from build123d import *

# Parameters (mm, degrees)
F0_R     = 20
F1_DEPTH = 5
F2_R     = 5
F3_DEPTH = 75
F4_R     = 4
F5_DEPTH = 3
F6_SIZE2 = 1
F6_SIZE  = 0.25
F7_R     = 4.99999
F9_D     = 2.75
F9_DEPTH = 7
F9_TIP   = 0.8261833512


# Not quite as in the source:
# - a fillet or chamfer is up to 0.001 mm smaller than in the source, because OpenCascade refuses the exact size


with BuildPart() as f1:
    # F0 (on Top) → F1 (new body)
    with BuildSketch(Plane.XY):
        Circle(F0_R)
    extrude(amount=F1_DEPTH)

    # F2 (on face) → F3 (join)
    with BuildSketch(Plane.XY.offset(5)):
        Circle(F2_R)
    extrude(amount=F3_DEPTH)

    # F4 (on face) → F5 (join)
    with BuildSketch(Plane.XY.offset(80)):
        Circle(F4_R)
    extrude(amount=F5_DEPTH)

    # F6
    f6_edges = [f1.edges().sort_by_distance(p)[0] for p in [
        (-4, 0, 83),
    ]]
    f6_side = f1.faces().sort_by_distance((0, 0, 83))[0]
    chamfer(f6_edges, length=F6_SIZE, length2=F6_SIZE2, reference=f6_side)

    # F7 (radius 5 in the source; OpenCascade refuses exactly that, so slightly less here)
    f7_edges = [f1.edges().sort_by_distance(p)[0] for p in [
        (-20, 0, 5),
        (-5, 0, 5),
    ]]
    fillet(f7_edges, radius=F7_R)

    # F9
    with Locations(Plane.XY.offset(83)):
        with Locations((0, 0)):
            Hole(F9_D / 2, depth=F9_DEPTH)
            with Locations((0, 0, -(F9_DEPTH + F9_TIP / 2))):  # 118° drill point
                Cone(0, F9_D / 2, F9_TIP, mode=Mode.SUBTRACT)


solid = f1.part
CAD build for the part. Positions are in the model's coordinates, mm. A direction names the side the tool comes from. Round coordinates to 2 decimals unless told otherwise and drop trailing zeros. Write each loop counter-clockwise with the first axis right and the second up, starting at its lowest first coordinate (ties: lowest second). Pieces come first, ordered by that corner, then holes. Notation, with made-up numbers: M -22.5,73 L 33.5,73 A17 ccw 33.5,89 Z; hole C 85.25,5.25 d7. An arc over 180 degrees is marked long. Put each result on its own line as item: value. Start each with the question number.
1) Pin check, flat tips, straight feed: pin 1 Ø8 at (x, z) = (-10.5, 36.5) entering from +Y; pin 2 Ø3 at (x, z) = (-3.5, 51) entering from +Y; pin 3 Ø1 at (x, y) = (8.5, -15.5) entering from +Z; pin 4 Ø10 at (x, y) = (9, -2.5) entering from +Z. Stop position of each tip, or through.
2) Drill centre lines: probe 1 along Y at (x, z) = (0, 78.5) (3 decimals); probe 2 along Z at (x, y) = (-7, -13); probe 3 along Y at (x, z) = (0, 81) (3 decimals). Where is each one in solid material? Low to high. Write a range as [from, to].
3) Saw through at A-A, the plane z = 36. Write the cut outline in (x, y).
4) Pull direction X, two halves, no side cores. Call faces 3 (the conical face through (0.23, 0.07, 75.32)), 4 (the cylindrical face through (-1.08, -4.88, 44.51)), 5 (the flat face through (0, 0, 0)), 6 (the cylindrical face through (0.3, -1.34, 79.45)): pulls with the +X half, pulls with the -X half, needs draft (parallel to the pull), parting line crosses it, or undercut.
5) 3-axis set-ups, long thin cutter, end or side, ignore diameter. For faces 1 (the flat face through (2, 0, 83)), 2 (the flat face through (10, -3, 5)): which of +Z, -Z, +X, -X, +Y, -Y reach the whole face in a straight line?
Resolved:
1. pin 1: through
1. pin 2: y = 4.58
1. pin 3: z = 4.5
1. pin 4: z = 80
2. probe 1: [-5, -1.375], [1.375, 5]
2. probe 2: [0, 5]
2. probe 3: [-4, -1.375], [1.375, 4]
3. outline: C 0,0 d10
4. face 3: undercut
4. face 4: parting line crosses it
4. face 5: needs draft
4. face 6: undercut
5. face 1: +Z, +X, -X, +Y, -Y
5. face 2: +Z
